Here's how the part is built. I have some questions about the finished solid (model axes, mm). A direction names the side the tool comes from. Give positions to 0.01 mm unless a question says otherwise; leave off trailing zeros. Loops run counter-clockwise (first coordinate to the right, second up) from the corner with the lowest first, then second, coordinate; pieces in that order, holes last. Notation, with made-up numbers: (-22, -24.75) - (-4, -24.75) arc R18 ccw to (-4, 10.25) - close; hole circle Ø1 at (-18.75, 47). An arc over 180 degrees is marked (long way). Use one line per item in the form item = value.
from build123d import *

# Parameters (mm, degrees)
F0_R   = 12.5
F0_R_2 = 6.35


with BuildPart() as f4:
    # F4: sweep along a path in F1, F3
    with BuildLine(Plane.XY) as f4_path:
        Line((0, 0), (0, -78.674))
        ThreePointArc((0, -78.674), (-22.3184632736, -132.5555367264), (-76.2, -154.874))
        Line((-76.2, -154.874), (-235.882, -154.874))
    with BuildLine(Plane.XZ.offset(154.874)) as f4_path_2:
        Line((-235.882, 0), (-258.9757317515, 0))
        ThreePointArc((-258.9757317515, 0), (-294.7448168404, -14.7276760951), (-309.7739216377, -50.371159374))
        Line((-309.7739216377, -50.371159374), (-310, -77.1512051091))
    # F0 (on Front) → F4 (sweep)
    with BuildSketch(Plane.XZ):
        Circle(F0_R)
        Circle(F0_R_2, mode=Mode.SUBTRACT)
    sweep(path=f4_path.line + f4_path_2.line)


solid = f4.part
(1) If I drill on probe 1 along Y at (x, z) = (-200, 0); probe 2 along Z at (x, y) = (-292.5, -158); probe 3 along X at (y, z) = (-68, 8.5), over which ranges is the centre line in solid material (lowest first)?
Geometry says:
probe_1 = -167.37 to -161.22, -148.52 to -142.37
probe_2 = -31.47 to -20.37, -5.54 to 2.42
probe_3 = -9.17 to 9.17
(2) Thinking about a two-plate mould opening in X: for faces 1 (the cylindrical face through (11.923, -39.888, 3.755)), 2 (the cylindrical face through (-315.24, -158.29, -63.9)), 3 (the flat face through (3, 0, 6)), which applies, pulls with the +X half, pulls with the -X half, needs draft (parallel to the pull), parting line crosses it, or undercut?
Geometry says:
face_1 = parting line crosses it
face_2 = undercut
face_3 = needs draft
(3) If we section it at B-B (x = -161): List the corners of the cut face in (y, z) for me.
Geometry says:
outline = circle Ø25 at (-154.87, 0); hole circle Ø12.7 at (-154.87, 0)
(4) If we section it at A-A (y = -59): List the corners of the cut face in (x, z) for me, plus the area to 3 significant figures.
Geometry says:
outline = circle Ø25 at (0, 0); hole circle Ø12.7 at (0, 0)
area = 364 mm²
(5) For faces 4 (the cylindrical face through (-1.38, -39.89, -6.2)), 5 (the cylindrical face through (-168.87, -160.93, 1.91)), which set-ups out of +Z, -Z, +X, -X, +Y, -Y let a thin tool reach every point of the face, with its end or its side?
Geometry says:
face_4 = +Y
face_5 = none
(6) For P1, Ø10, axis at y = -154.874, z = 0, coming from the -X side; P2, Ø8, axis at y = -117.5, z = -0.5, coming from the -X side, each with a flat end and sliding along its axis, tell me the tip position at first contact or that it passes through.
Geometry says:
P1 = -302.67
P2 = -29.04
